Autodesk Fusion 360 part; units mm, degrees
sketch "Sketch1" plane through (0, 0, 0) normal (0, 1, 0) x (1, 0, 0)
  line L0 (0, 12.575) -> (27.15, 12.575) construction
  line L1 (27.15, 12.575) -> (27.15, -8.575)
  line L2 (23.15, -12.575) -> (0, -12.575)
  line L3 (27.15, 12.575) -> (33.15, 12.575)
  line L4 (33.15, 12.575) -> (33.15, 6.575)
  line L5 (33.15, 6.575) -> (27.15, 6.575)
  line L6 (27.15, 6.575) -> (27.15, 12.575)
  line L7 (0, -12.575) -> (0, 12.575) construction
  circle A0 centre (30.15, 9.575) radius 1.425
  line L8 (27.15, 6.575) -> (33.15, 12.575) construction
  arc A1 (23.15, -12.575) -> (27.15, -8.575) centre (23.15, -8.575) ccw
  line L9 (-27.15, 12.575) -> (-27.15, -8.575)
  line L10 (-33.15, 6.575) -> (-27.15, 6.575)
  circle A2 centre (-30.15, 9.575) radius 1.425
  line L11 (-27.15, 12.575) -> (-33.15, 12.575)
  line L12 (-33.15, 12.575) -> (-33.15, 6.575)
  line L13 (-23.15, -12.575) -> (0, -12.575)
  arc A3 (-27.15, -8.575) -> (-23.15, -12.575) centre (-23.15, -8.575) ccw
  line L14 (-27.15, 0) -> (27.15, 0) construction
  line L15 (-27.15, 12.575) -> (-27.15, 22.575)
  line L16 (-27.15, 22.575) -> (27.15, 22.575)
  line L17 (27.15, 22.575) -> (27.15, 12.575)
  line L18 (-10, -8.575) -> (-10, 18.575)
  line L19 (-10, 18.575) -> (-8, 18.575)
  line L20 (-8, 18.575) -> (-8, -8.575)
  line L21 (-8, -8.575) -> (-10, -8.575)
  line L22 (-16, -8.575) -> (-16, 18.575)
  line L23 (-16, 18.575) -> (-14, 18.575)
  line L24 (-14, 18.575) -> (-14, -8.575)
  line L25 (-14, -8.575) -> (-16, -8.575)
  line L26 (-22, -8.575) -> (-22, 18.575)
  line L27 (-22, 18.575) -> (-20, 18.575)
  line L28 (-20, 18.575) -> (-20, -8.575)
  line L29 (-20, -8.575) -> (-22, -8.575)
  line L30 (-4, 18.075) -> (4, 18.075)
  line L31 (-4, 18.075) -> (-8.5, 22.575)
  line L32 (4, 18.075) -> (8.5, 22.575)
  line L33 (20, -8.575) -> (22, -8.575)
  line L34 (14, -8.575) -> (16, -8.575)
  line L35 (8, 18.575) -> (8, -8.575)
  line L36 (22, 18.575) -> (20, 18.575)
  line L37 (10, 18.575) -> (8, 18.575)
  line L38 (8, -8.575) -> (10, -8.575)
  line L39 (16, -8.575) -> (16, 18.575)
  line L40 (22, -8.575) -> (22, 18.575)
  line L41 (14, 18.575) -> (14, -8.575)
  line L42 (16, 18.575) -> (14, 18.575)
  line L43 (10, -8.575) -> (10, 18.575)
  line L44 (20, 18.575) -> (20, -8.575)
  line L45 (-4, 15.075) -> (-2, 15.075)
  line L46 (-2, 15.075) -> (-2, -8.575)
  line L47 (-2, -8.575) -> (-4, -8.575)
  line L48 (-4, -8.575) -> (-4, 15.075)
  line L49 (4, 15.075) -> (2, 15.075)
  line L50 (2, 15.075) -> (2, -8.575)
  line L51 (4, -8.575) -> (4, 15.075)
  line L52 (2, -8.575) -> (4, -8.575)
  point P0 (23.15, -8.575)
  point P1 (0, 18.075)
  dimension "d1" = 6
  dimension "d2" = 6
  dimension "d4" = 33.15
  dimension "d5" = 2.85
  dimension "d6" = 4
  dimension "d16" = 10
  dimension "d18" = 25.15
  dimension "d25" = 4.5
  dimension "d26" = 45
  dimension "d27" = 45
  dimension "d28" = 2
  dimension "d29" = 8
  dimension "d30" = 27.15
  dimension "d31" = 4
  dimension "d32" = 4
  dimension "d33" = 4
  dimension "d34" = 8
  dimension "d35" = 4
  dimension "d36" = 3
extrude "Extrude1" add sketch "Sketch1" along normal blind 2 contours L1 L3 L4 L5 L6 | L1 L2 L6 A1 L9 L13 A3 L15 L16 L17 L30 L31 L32 | L9 L10 L11 L12
Geometry: final body of the model. Coordinates: model frame, mm. A direction names the side the tool comes from. Round coordinates to 2 decimals unless told otherwise and drop trailing zeros. Loops run counter-clockwise (first coordinate to the right, second up) from the corner with the lowest first, then second, coordinate; pieces in that order, holes last. Notation, with made-up numbers: (21.5, 55) - (78.5, 55) arc R12 cw to (78.5, 77) - close; hole circle Ø2 at (2, 84). An arc over 180 degrees is marked (long way). Write each question's results on one line, items separated by ' | '. Start each with the question number.
1) Access query for faces 1 (the face through (-6.219, 0.986, -20.294)), 2 (the face through (-30, 1, -6.575)), 3 (the face through (-27.15, 1, -18)), 4 (the face through (3, 1, 8.575)). Directions: +Z, -Z, +X, -X, +Y, -Y. A direction counts if a zero-diameter tool reaches every point of the face in a straight line with its end or side. Return the directions, or none.
2) First-contact query: P1, Ø1, axis at y = 0.5, z = 3.5, coming from the +X side; P2, Ø0.6, axis at y = 1, z = -1.5, coming from the -X side; P3, Ø12, axis at x = -23.5, z = -14, coming from the -Y side. Flat tips, straight axial feed; report the tip coordinate or a pass-through.
3) Line query: probe 1 along Z at (x, y) = (-30.15, 1.2) (3 decimals); probe 2 along Z at (x, y) = (-1, 1.35) (3 decimals); probe 3 along Z at (x, y) = (-5, 1.8) (3 decimals). Output: solid intervals per line, ascending. Write a range as [from, to].
4) Cut plane B-B on x = 30.15. Return loops of the section in (y, z) (3 decimals), then the cut area to 3 significant figures.
5) Cut plane C-C on z = 5. Count the separate pieces of the cut face and the enclosed holes in it, then the cut area to 3 significant figures.
6) Mould query, pull axis X, two halves, no side actions, for faces 5 (the face through (29.02, 0.99, -10.44)), 6 (the face through (26.01, 0.99, 11.37)), 7 (the face through (30, 1, -12.575)). Classes: released by +X, released by -X, zero draft, split by the parting line, or undercut.
7) Cut plane A-A on z = -17. Return loops of the section in (x, y).
Verdict:
1) face 1: -Z, +Y, -Y | face 2: +Z, -X, +Y, -Y | face 3: -Z, -X, +Y, -Y | face 4: +Y, -Y
2) P1: stops at x = 27.15 | P2: stops at x = -27.15 | P3: stops at y = 0
3) probe 1: z = [-12.575, -11], [-8.15, -6.575] | probe 2: z = [-18.075, 12.575] | probe 3: z = [-19.075, 12.575]
4) outline: (0, -12.575) - (2, -12.575) - (2, -11) - (0, -11) - close; (0, -8.15) - (2, -8.15) - (2, -6.575) - (0, -6.575) - close | area: 6.30 mm2
5) separate pieces: 9 | enclosed holes: 0 | area: 76.6 mm2
6) face 5: undercut | face 6: released by +X | face 7: zero draft
7) outline: (-27.15, 0) - (-22, 0) - (-22, 2) - (-27.15, 2) - close; (-20, 0) - (-16, 0) - (-16, 2) - (-20, 2) - close; (-14, 0) - (-10, 0) - (-10, 2) - (-14, 2) - close; (-8, 0) - (8, 0) - (8, 2) - (-8, 2) - close; (10, 0) - (14, 0) - (14, 2) - (10, 2) - close; (16, 0) - (20, 0) - (20, 2) - (16, 2) - close; (22, 0) - (27.15, 0) - (27.15, 2) - (22, 2) - close
